```python
from build123d import *

# Parameters (mm, degrees)
SKETCH1_W           = 80
SKETCH1_H           = 40
BOSS_EXTRUDE1_DEPTH = 5
CUT_EXTRUDE4_REACH  = 91.582
CUT_EXTRUDE5_REACH  = 91.582
SKETCH11_R          = 2.525
FILLET1_R           = 3
CUT_EXTRUDE9_REACH  = 91.582
SKETCH19_R          = 1.525
SKETCH19_R_2        = 6


with BuildPart() as part:
    # Sketch1 → Boss-Extrude1 (new body)
    with BuildSketch(Plane.XY):
        with Locations((40, 20)):
            Rectangle(SKETCH1_W, SKETCH1_H)
    extrude(amount=BOSS_EXTRUDE1_DEPTH)

    # Sketch10 → Cut-Extrude4 (cut, up to next)
    with BuildSketch(Plane.XY.offset(5), mode=Mode.PRIVATE) as cut_extrude4_sk1:
        with BuildLine():
            ThreePointArc((20, 0), (5.857864376, 5.857864376), (0, 20))
            Line((0, 20), (0, 0))
            Line((0, 0), (20, 0))
        make_face()
    cut_extrude4_tool1 = extrude(cut_extrude4_sk1.sketch, amount=-CUT_EXTRUDE4_REACH, mode=Mode.PRIVATE) & part.part
    # Sketch10 → Cut-Extrude4 (cut, up to next)
    with BuildSketch(Plane.XY.offset(5), mode=Mode.PRIVATE) as cut_extrude4_sk2:
        with BuildLine():
            Line((20, 40), (0, 40))
            Line((0, 40), (0, 20))
            ThreePointArc((0, 20), (5.857864376, 34.142135624), (20, 40))
        make_face()
    cut_extrude4_tool2 = extrude(cut_extrude4_sk2.sketch, amount=-CUT_EXTRUDE4_REACH, mode=Mode.PRIVATE) & part.part
    add(cut_extrude4_tool1.solids().sort_by_distance((4.467359, 4.467359, 5))[0], mode=Mode.SUBTRACT)
    add(cut_extrude4_tool2.solids().sort_by_distance((4.467359, 35.532641, 5))[0], mode=Mode.SUBTRACT)

    # Sketch11 → Cut-Extrude5 (cut, up to next)
    with BuildSketch(Plane.XY.offset(5), mode=Mode.PRIVATE) as cut_extrude5_sk1:
        with Locations((55, 30)):
            Circle(SKETCH11_R)
    cut_extrude5_tool1 = extrude(cut_extrude5_sk1.sketch, amount=-CUT_EXTRUDE5_REACH, mode=Mode.PRIVATE) & part.part
    # Sketch11 → Cut-Extrude5 (cut, up to next)
    with BuildSketch(Plane.XY.offset(5), mode=Mode.PRIVATE) as cut_extrude5_sk2:
        with Locations((70, 30)):
            Circle(SKETCH11_R)
    cut_extrude5_tool2 = extrude(cut_extrude5_sk2.sketch, amount=-CUT_EXTRUDE5_REACH, mode=Mode.PRIVATE) & part.part
    # Sketch11 → Cut-Extrude5 (cut, up to next)
    with BuildSketch(Plane.XY.offset(5), mode=Mode.PRIVATE) as cut_extrude5_sk3:
        with Locations((55, 10)):
            Circle(SKETCH11_R)
    cut_extrude5_tool3 = extrude(cut_extrude5_sk3.sketch, amount=-CUT_EXTRUDE5_REACH, mode=Mode.PRIVATE) & part.part
    # Sketch11 → Cut-Extrude5 (cut, up to next)
    with BuildSketch(Plane.XY.offset(5), mode=Mode.PRIVATE) as cut_extrude5_sk4:
        with Locations((70, 10)):
            Circle(SKETCH11_R)
    cut_extrude5_tool4 = extrude(cut_extrude5_sk4.sketch, amount=-CUT_EXTRUDE5_REACH, mode=Mode.PRIVATE) & part.part
    add(cut_extrude5_tool1.solids().sort_by_distance((55, 30, 5))[0], mode=Mode.SUBTRACT)
    add(cut_extrude5_tool2.solids().sort_by_distance((70, 30, 5))[0], mode=Mode.SUBTRACT)
    add(cut_extrude5_tool3.solids().sort_by_distance((55, 10, 5))[0], mode=Mode.SUBTRACT)
    add(cut_extrude5_tool4.solids().sort_by_distance((70, 10, 5))[0], mode=Mode.SUBTRACT)

    # Fillet1
    fillet1_edges = [part.edges().sort_by_distance(p)[0] for p in [
        (80, 40, 2.5),
        (80, 0, 2.5),
    ]]
    fillet(fillet1_edges, radius=FILLET1_R)

    # Sketch19 → Cut-Extrude9 (cut, up to next)
    with BuildSketch(Plane.XY.offset(5), mode=Mode.PRIVATE) as cut_extrude9_sk1:
        with Locations((20, 35.5)):
            Circle(SKETCH19_R)
    cut_extrude9_tool1 = extrude(cut_extrude9_sk1.sketch, amount=-CUT_EXTRUDE9_REACH, mode=Mode.PRIVATE) & part.part
    # Sketch19 → Cut-Extrude9 (cut, up to next)
    with BuildSketch(Plane.XY.offset(5), mode=Mode.PRIVATE) as cut_extrude9_sk2:
        with Locations((33.423393759, 27.75)):
            Circle(SKETCH19_R)
    cut_extrude9_tool2 = extrude(cut_extrude9_sk2.sketch, amount=-CUT_EXTRUDE9_REACH, mode=Mode.PRIVATE) & part.part
    # Sketch19 → Cut-Extrude9 (cut, up to next)
    with BuildSketch(Plane.XY.offset(5), mode=Mode.PRIVATE) as cut_extrude9_sk3:
        with Locations((33.423393759, 12.25)):
            Circle(SKETCH19_R)
    cut_extrude9_tool3 = extrude(cut_extrude9_sk3.sketch, amount=-CUT_EXTRUDE9_REACH, mode=Mode.PRIVATE) & part.part
    # Sketch19 → Cut-Extrude9 (cut, up to next)
    with BuildSketch(Plane.XY.offset(5), mode=Mode.PRIVATE) as cut_extrude9_sk4:
        with Locations((20, 4.5)):
            Circle(SKETCH19_R)
    cut_extrude9_tool4 = extrude(cut_extrude9_sk4.sketch, amount=-CUT_EXTRUDE9_REACH, mode=Mode.PRIVATE) & part.part
    # Sketch19 → Cut-Extrude9 (cut, up to next)
    with BuildSketch(Plane.XY.offset(5), mode=Mode.PRIVATE) as cut_extrude9_sk5:
        with Locations((6.576606241, 12.25)):
            Circle(SKETCH19_R)
    cut_extrude9_tool5 = extrude(cut_extrude9_sk5.sketch, amount=-CUT_EXTRUDE9_REACH, mode=Mode.PRIVATE) & part.part
    # Sketch19 → Cut-Extrude9 (cut, up to next)
    with BuildSketch(Plane.XY.offset(5), mode=Mode.PRIVATE) as cut_extrude9_sk6:
        with Locations((6.576606241, 27.75)):
            Circle(SKETCH19_R)
    cut_extrude9_tool6 = extrude(cut_extrude9_sk6.sketch, amount=-CUT_EXTRUDE9_REACH, mode=Mode.PRIVATE) & part.part
    # Sketch19 → Cut-Extrude9 (cut, up to next)
    with BuildSketch(Plane.XY.offset(5), mode=Mode.PRIVATE) as cut_extrude9_sk7:
        with Locations((13, 20)):
            Circle(SKETCH19_R_2)
    cut_extrude9_tool7 = extrude(cut_extrude9_sk7.sketch, amount=-CUT_EXTRUDE9_REACH, mode=Mode.PRIVATE) & part.part
    add(cut_extrude9_tool1.solids().sort_by_distance((20, 35.5, 5))[0], mode=Mode.SUBTRACT)
    add(cut_extrude9_tool2.solids().sort_by_distance((33.423394, 27.75, 5))[0], mode=Mode.SUBTRACT)
    add(cut_extrude9_tool3.solids().sort_by_distance((33.423394, 12.25, 5))[0], mode=Mode.SUBTRACT)
    add(cut_extrude9_tool4.solids().sort_by_distance((20, 4.5, 5))[0], mode=Mode.SUBTRACT)
    add(cut_extrude9_tool5.solids().sort_by_distance((6.576606, 12.25, 5))[0], mode=Mode.SUBTRACT)
    add(cut_extrude9_tool6.solids().sort_by_distance((6.576606, 27.75, 5))[0], mode=Mode.SUBTRACT)
    add(cut_extrude9_tool7.solids().sort_by_distance((13, 20, 5))[0], mode=Mode.SUBTRACT)


solid = part.part
```
Can you work these out from the model? Positions are in its coordinate system, mm. Give positions to 0.01 mm unless a question says otherwise; leave off trailing zeros. Order: outer loops, then holes, each group sorted by start corner. A loop starts at its lowest first (then second) coordinate and runs counter-clockwise, first axis right, second up. Notation, with made-up numbers: M -14,69 L -5,69 A15 ccw -5,88 Z; hole C -2,-12.5 d8. An arc over 180 degrees is marked long. One line per item, written item: value.
1) We'd pull the mould along Y, two halves only. Please class faces 1 (the face through (79.1, 0.86, 2.54)), 2 (the face through (80, 20, 2)), 3 (the face through (71.165, 27.76, 2.535)): released by +Y, released by -Y, zero draft, split by the parting line, or undercut.
Answer sheet:
face 1: released by -Y
face 2: zero draft
face 3: undercut
2) I want a section at C-C, the plane y = 24.5. List the corners of the cut face in (x, z) for me, plus the area to 3 significant figures.
Answer sheet:
outline: M 0.51,0 L 9.03,0 L 9.03,5 L 0.51,5 Z; M 16.97,0 L 80,0 L 80,5 L 16.97,5 Z
area: 358 mm^2
3) I want a section at B-B, the plane z = 0.75. Count the separate pieces of the cut face and the enclosed holes in it, plus the area to 3 significant figures.
Answer sheet:
separate pieces: 1
enclosed holes: 11
area: 2,790 mm^2
4) Please list where these lines run through material, in increasing order: line 1 along Y through (x, z) = (69.5, 1.15) (3 decimals); line 2 along X through (y, z) = (13.5, 3.7); line 3 along X through (y, z) = (10.5, 1.9) (3 decimals).
Answer sheet:
line 1: y = 0 to 7.525, 12.475 to 27.525, 32.475 to 40
line 2: x = 1.09 to 5.7, 7.45 to 32.55, 34.3 to 80
line 3: x = 2.4 to 52.525, 57.475 to 67.525, 72.475 to 80
5) I want a section at A-A, the plane x = 70. List the corners of the cut face in (y, z) for me (3 decimals), plus the area to 4 significant figures.
Answer sheet:
outline: M 0,0 L 7.475,0 L 7.475,5 L 0,5 Z; M 12.525,0 L 27.475,0 L 27.475,5 L 12.525,5 Z; M 32.525,0 L 40,0 L 40,5 L 32.525,5 Z
area: 149.5 mm^2
6) I want a section at D-D, the plane y = 31. List the corners of the cut face in (x, z) for me.
Answer sheet:
outline: M 3.3,0 L 52.68,0 L 52.68,5 L 3.3,5 Z; M 57.32,0 L 67.68,0 L 67.68,5 L 57.32,5 Z; M 72.32,0 L 80,0 L 80,5 L 72.32,5 Z
7) For P1, Ø2.5, axis at x = 33.42, y = 12.25, coming from the -Z side; P2, Ø3.5, axis at x = 6.58, y = 12.25, coming from the +Z side, each with a flat end and sliding along its axis, tell me the tip position at first contact or that it passes through.
Answer sheet:
P1: passes through
P2: stops at z = 5
